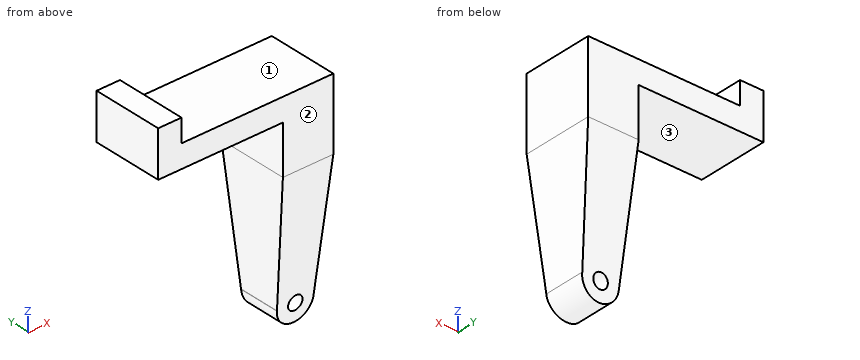
```python
from build123d import *

# Parameters (mm, degrees)
F0_W     = 6.4516
F0_H     = 19.6342
F0_W_2   = 28.067
F0_W_3   = 13.97
F1_DEPTH = 6.35
F2_DEPTH = 6.35
F3_DEPTH = 60.96
F5_DEPTH = 19.6352
F4_R     = 1.9939
F6_DEPTH = 19.6352
F8_DEPTH = 48.4896


with BuildPart() as f1:
    # F0 (on Top) → F1 (new body)
    with BuildSketch(Plane.XY):
        with Locations((-22.536153, 17.688083)):
            Rectangle(F0_W, F0_H)
        with Locations((-5.276853, 17.688083)):
            Rectangle(F0_W_2, F0_H)
        with Locations((15.741647, 17.688083)):
            Rectangle(F0_W_3, F0_H)
    extrude(amount=-F1_DEPTH)

    # F0 (on Top) → F2 (join)
    with BuildSketch(Plane.XY):
        with Locations((-22.536153, 17.688083)):
            Rectangle(F0_W, F0_H)
    extrude(amount=F2_DEPTH)

    # F0 (on Top) → F3 (join)
    with BuildSketch(Plane.XY):
        with Locations((15.741647, 17.688083)):
            Rectangle(F0_W_3, F0_H)
    extrude(amount=-F3_DEPTH)

    # F4 (on face) → F5 (cut, through all)
    with BuildSketch(Plane(origin=(0, 27.505183, 0), x_dir=(-1, 0, 0), z_dir=(0, 1, 0))):
        with BuildLine():
            ThreePointArc((-10.662622, -55.478505), (-10.66189, -55.528265), (-10.661647, -55.578031))
            ThreePointArc((-10.661647, -55.578031), (-15.791412, -60.657787), (-20.820672, -55.478505))
            Line((-20.820672, -55.478505), (-22.726647, -19.884773))
            Line((-22.726647, -19.884773), (-22.726647, -60.96))
            Line((-22.726647, -60.96), (-8.756647, -60.96))
            Line((-8.756647, -60.96), (-8.756647, -19.884773))
            Line((-8.756647, -19.884773), (-10.662622, -55.478505))
        make_face()
    extrude(amount=-F5_DEPTH, mode=Mode.SUBTRACT)

    # F4 (on face) → F6 (cut, through all)
    with BuildSketch(Plane(origin=(0, 27.505183, 0), x_dir=(-1, 0, 0), z_dir=(0, 1, 0))):
        with Locations((-15.741647, -55.578031)):
            Circle(F4_R)
    extrude(amount=-F6_DEPTH, mode=Mode.SUBTRACT)

    # F7 (on face) → F8 (cut, through all)
    with BuildSketch(Plane.YZ.offset(22.726647)):
        Polygon((22.828814, -60.658031), (27.505183, -60.658031), (27.505183, -55.478505), (27.505183, -19.884773), align=None)
        Polygon((7.870983, -60.658031), (12.547351, -60.658031), (7.870983, -19.884773), (7.870983, -55.478505), align=None)
    extrude(amount=-F8_DEPTH, mode=Mode.SUBTRACT)


solid = f1.part
```
Geometry: final body of the model. Coordinates: model frame, mm. Face numbers are marked on the shaded views. A direction names the side the tool comes from. Give positions to 0.01 mm unless a question says otherwise; leave off trailing zeros. Order: outer loops, then holes, each group sorted by start corner. A loop starts at its lowest first (then second) coordinate and runs counter-clockwise, first axis right, second up. Notation, with made-up numbers: (34.25, 39.25) -> (63.25, 39.25) arc R21 cw to (63.25, 77.25) -> close; hole circle Ø5 at (-11, -0.5). An arc over 180 degrees is marked (long way). Write each question's results on one line, items separated by ' | '. Start each with the question number.
1) Section A-A (y = 17.25). Return loops of the section in (x, z), then the cut area to 3 significant figures.
2) First-contact query: pin 1 (8 mm diameter, centred on x = -12.5, y = 24, fed in from -Z); pin 2 (6 mm diameter, centred on x = 6.5, y = 13, fed in from +Z); pin 3 (10 mm diameter, centred on x = 16, z = -53, fed in from +Y); pin 4 (3.5 mm diameter, centred on x = 15.74, z = -55.58, fed in from -Y). Flat tips, straight axial feed; report the tip coordinate or a pass-through.
3) Line query: line 1 (X direction, y = 24.75, z = -15); line 2 (Z direction, x = -5, y = 11.75); line 3 (Z direction, x = -20, y = 23.75). Output: solid intervals per line, ascending. Write a range as from..to.
4) Section B-B (x = -5). Return loops of the section in (y, z), then the cut area to 3 significant figures.
5) Section C-C (z = -12.5). Return loops of the section in (x, y), then the cut area to 3 significant figures.
6) Set-up query: the marked faces 1, 2 and 3. Return all of +Z, -Z, +X, -X, +Y, -Y with unobstructed straight access to the full face (end or side cutting, diameter ignored); none if empty.
Calculated:
1) outline: (-25.76, -6.35) -> (8.76, -6.35) -> (8.76, -19.88) -> (10.66, -55.48) arc R5.06 ccw to (10.66, -55.58) arc R5.08 ccw (long way) to (20.82, -55.48) -> (22.73, -19.88) -> (22.73, 0) -> (-19.31, 0) -> (-19.31, 6.35) -> (-25.76, 6.35) -> close; hole circle Ø3.99 at (15.74, -55.58) | area: 996 mm2
2) pin 1: z = -6.35 | pin 2: z = 0 | pin 3: y = 24.28 | pin 4: through
3) line 1: 8.76..22.73 | line 2: -6.35..0 | line 3: -6.35..6.35
4) outline: (7.87, -6.35) -> (27.51, -6.35) -> (27.51, 0) -> (7.87, 0) -> close | area: 125 mm2
5) outline: (8.76, 7.87) -> (22.73, 7.87) -> (22.73, 27.51) -> (8.76, 27.51) -> close | area: 274 mm2
6) face 1: +Z, +X, +Y, -Y | face 2: +Z, -Z, +X, -X, -Y | face 3: -Z, -X, +Y, -Y
